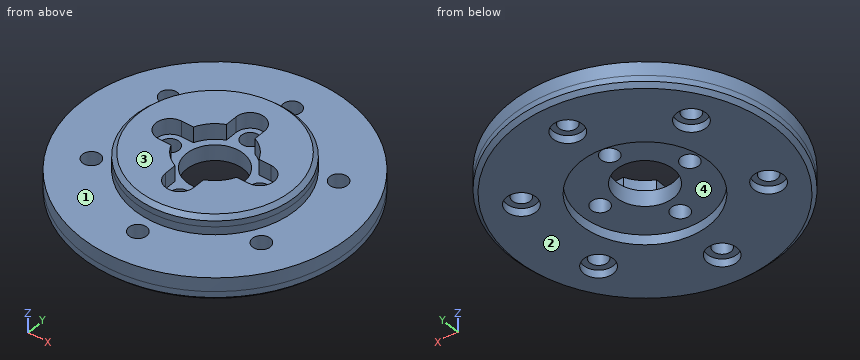
from build123d import *
from build123d.topology import SkipClean

# Parameters (mm, degrees)
SKETCH1_R               = 34.1
BOSS_EXTRUDE1_DEPTH     = 1.75
SKETCH4_R               = 28.5
BOSS_EXTRUDE2_DEPTH     = 2
SKETCH5_R               = 34.1
SKETCH5_R_2             = 16.25
BOSS_EXTRUDE3_DEPTH     = 2.5
CUT_EXTRUDE2_DEPTH      = 49.596501932
CUT_EXTRUDE2_DEPTH_BACK = 49.596501932
SKETCH3_R               = 2.25
CUT_EXTRUDE1_DEPTH      = 49.596501932
CUT_EXTRUDE1_DEPTH_BACK = 49.596501932
SKETCH2_R               = 7.25
SKETCH7_R               = 20.5
SKETCH7_R_2             = 2.25
SKETCH7_R_3             = 7.25
BOSS_EXTRUDE4_DEPTH     = 2.5
BOSS_EXTRUDE5_START     = 2
SKETCH8_R               = 34.1
SKETCH8_R_2             = 28.5
BOSS_EXTRUDE5_DEPTH     = 2
SKETCH10_R              = 34.1
SKETCH10_R_2            = 20.5
CUT_EXTRUDE4_DEPTH      = 2
CUT_EXTRUDE5_DEPTH      = 4
SKETCH6_R               = 2.25
CUT_EXTRUDE3_DEPTH      = 50.354533733
SKETCH12_R              = 3.75
CUT_EXTRUDE6_DEPTH      = 2
CIRPATTERN1_COUNT       = 6
CHAMFER1_SIZE           = 1


with BuildPart() as part:
    # Sketch1 → Boss-Extrude1 (new, symmetric)
    with BuildSketch(Plane.XY):
        Circle(SKETCH1_R)
    extrude(amount=BOSS_EXTRUDE1_DEPTH, both=True)

    # Sketch4 → Boss-Extrude2 (add)
    with BuildSketch(Plane.XY.offset(1.75)):
        Circle(SKETCH4_R)
    extrude(amount=BOSS_EXTRUDE2_DEPTH)

    # Sketch5 → Boss-Extrude3 (add)
    with BuildSketch(Plane(origin=(0, 0, -1.75), x_dir=(-1, 0, 0), z_dir=(0, 0, -1))):
        Circle(SKETCH5_R)
        Circle(SKETCH5_R_2, mode=Mode.SUBTRACT)
    extrude(amount=BOSS_EXTRUDE3_DEPTH)

    # Sketch3 → Cut-Extrude2 (cut, two sides: drawn at the far end of the back side and taken through both)
    with BuildSketch(Plane.XY.offset(1.75).offset(-CUT_EXTRUDE2_DEPTH_BACK)):
        with Locations((0, 11.3137085)):
            Circle(SKETCH3_R)
        with Locations((11.3137085, 0)):
            Circle(SKETCH3_R)
        with Locations((0, -11.3137085)):
            Circle(SKETCH3_R)
        with Locations((-11.3137085, 0)):
            Circle(SKETCH3_R)
    extrude(amount=CUT_EXTRUDE2_DEPTH + CUT_EXTRUDE2_DEPTH_BACK, mode=Mode.SUBTRACT)

    # Sketch2 → Cut-Extrude1 (cut, two sides: drawn at the far end of the back side and taken through both)
    with BuildSketch(Plane.XY.offset(1.75).offset(-CUT_EXTRUDE1_DEPTH_BACK)):
        Circle(SKETCH2_R)
    extrude(amount=CUT_EXTRUDE1_DEPTH + CUT_EXTRUDE1_DEPTH_BACK, mode=Mode.SUBTRACT)

    # Sketch7 → Boss-Extrude4 (add)
    with BuildSketch(Plane.XY.offset(3.75)):
        Circle(SKETCH7_R)
        with Locations((0, -11.3137085)):
            Circle(SKETCH7_R_2, mode=Mode.SUBTRACT)
        with Locations((11.3137085, 0)):
            Circle(SKETCH7_R_2, mode=Mode.SUBTRACT)
        with Locations((0, 11.3137085)):
            Circle(SKETCH7_R_2, mode=Mode.SUBTRACT)
        with Locations((-11.3137085, 0)):
            Circle(SKETCH7_R_2, mode=Mode.SUBTRACT)
        Circle(SKETCH7_R_3, mode=Mode.SUBTRACT)
    extrude(amount=BOSS_EXTRUDE4_DEPTH)

    # Sketch8 → Boss-Extrude5 (add)
    with SkipClean():  # the faces are left unmerged after this step: merging them gives an invalid solid
        with BuildSketch(Plane.XY.offset(1.75).offset(BOSS_EXTRUDE5_START)):
            with Locations(Location((0, 0, 0), (0, 0, 180))):
                Circle(SKETCH8_R)
            Circle(SKETCH8_R_2, mode=Mode.SUBTRACT)
        extrude(amount=-BOSS_EXTRUDE5_DEPTH)

    # Sketch10 → Cut-Extrude4 (cut)
    with BuildSketch(Plane.XY.offset(3.75)):
        with Locations(Location((0, 0, 0), (0, 0, 180))):
            Circle(SKETCH10_R)
        Circle(SKETCH10_R_2, mode=Mode.SUBTRACT)
    extrude(amount=-CUT_EXTRUDE4_DEPTH, mode=Mode.SUBTRACT)

    # Sketch11 → Cut-Extrude5 (cut)
    with BuildSketch(Plane.XY.offset(6.25)):
        with BuildLine():
            Line((-11.3137085, 3.6), (-8.248636251, 3.6))
            ThreePointArc((-8.248636251, 3.6), (-6.363961031, 6.363961031), (-3.6, 8.248636251))
            Line((-3.6, 8.248636251), (-3.6, 11.3137085))
            ThreePointArc((-3.6, 11.3137085), (0, 14.9137085), (3.6, 11.3137085))
            Line((3.6, 11.3137085), (3.6, 8.248636251))
            ThreePointArc((3.6, 8.248636251), (6.363961031, 6.363961031), (8.248636251, 3.6))
            Line((8.248636251, 3.6), (11.3137085, 3.6))
            ThreePointArc((11.3137085, 3.6), (14.9137085, 0), (11.3137085, -3.6))
            Line((11.3137085, -3.6), (8.248636251, -3.6))
            ThreePointArc((8.248636251, -3.6), (6.363961031, -6.363961031), (3.6, -8.248636251))
            Line((3.6, -8.248636251), (3.6, -11.3137085))
            ThreePointArc((3.6, -11.3137085), (0, -14.9137085), (-3.6, -11.3137085))
            Line((-3.6, -11.3137085), (-3.6, -8.248636251))
            ThreePointArc((-3.6, -8.248636251), (-6.363961031, -6.363961031), (-8.248636251, -3.6))
            Line((-8.248636251, -3.6), (-11.3137085, -3.6))
            ThreePointArc((-11.3137085, -3.6), (-14.9137085, 0), (-11.3137085, 3.6))
        make_face()
    extrude(amount=-CUT_EXTRUDE5_DEPTH, mode=Mode.SUBTRACT)

    # Sketch6 → Cut-Extrude3 (cut, symmetric)
    with BuildSketch(Plane.XY.offset(-4.25)):
        with Locations((0, 24.75)):
            Circle(SKETCH6_R)
    cut_extrude3 = extrude(amount=CUT_EXTRUDE3_DEPTH, both=True, mode=Mode.SUBTRACT)

    # Sketch12 → Cut-Extrude6 (cut)
    with BuildSketch(Plane(origin=(0, 0, -4.25), x_dir=(-1, 0, 0), z_dir=(0, 0, -1))):
        with Locations((0, 24.75)):
            Circle(SKETCH12_R)
    cut_extrude6 = extrude(amount=-CUT_EXTRUDE6_DEPTH, mode=Mode.SUBTRACT)

    # CirPattern1: Cut-Extrude3, Cut-Extrude6 ×6 about axis
    cirpattern1_axis = Axis((0, 0, 0), (0, 0, 1))
    add([cut_extrude3.rotate(cirpattern1_axis, i * 360 / CIRPATTERN1_COUNT) for i in range(1, CIRPATTERN1_COUNT)], mode=Mode.SUBTRACT)
    add([cut_extrude6.rotate(cirpattern1_axis, i * 360 / CIRPATTERN1_COUNT) for i in range(1, CIRPATTERN1_COUNT)], mode=Mode.SUBTRACT)

    # Chamfer1
    chamfer1_edges = [part.edges().sort_by_distance(p)[0] for p in [
        (34.1, 0, -4.25),
        (-20.5, 0, 6.25),
    ]]
    chamfer(chamfer1_edges, length=CHAMFER1_SIZE)


solid = part.part
Could you check a few things on this model? Use its own coordinates, in mm. Face numbers are marked on the shaded views. A direction names the side the tool comes from. Give positions to 0.01 mm unless a question says otherwise; leave off trailing zeros. Return JSON: item names as keys, results as strings.
1. I need wall thicknesses on line 1 (Y direction, x = 0, z = 1.2); line 2 (X direction, y = 11, z = -1.25); line 3 (Z direction, x = -13.5, y = 17.5). Which ranges of each line are inside material? Lowest first, please. Write a range as from..to.
Answer list:
{"line 1": "y = -34.1..-27, -22.5..-13.56, -9.06..-7.25, 7.25..9.06, 13.56..22.5, 27..34.1", "line 2": "x = -32.28..-23.22, -19.65..-2.23, 2.23..19.65, 23.22..32.28", "line 3": "z = -4.25..1.75"}
2. Imagine slicing it at A-A on y = 0. Give the number of separate pieces and of enclosed holes in the cut face, then the cut area to 3 significant figures.
Answer list:
{"separate pieces": "4", "enclosed holes": "0", "area": "297 mm2"}
3. On a 3-axis mill with a long thin cutter (end or side, diameter ignored), from which of +Z, -Z, +X, -X, +Y, -Y can I reach the whole of each face in a straight line? I mean the marked faces 1 and 2. Say none if no direction works.
Answer list:
{"face 1": "+Z", "face 2": "-Z, +X, -X, +Y, -Y"}
4. Thinking about a two-plate mould opening in Y: for the marked faces 3 and 4, which applies, pulls with the +Y half, pulls with the -Y half, needs draft (parallel to the pull), parting line crosses it, or undercut?
Answer list:
{"face 3": "needs draft", "face 4": "undercut"}
5. For pin 1 Ø3.5 at (y, z) = (-9.5, 5) entering from +X; pin 2 Ø6 at (x, y) = (22, 25.5) entering from -Z; pin 3 Ø6 at (x, y) = (-21.5, -12.5) entering from -Z; pin 4 Ø6 at (x, z) = (-26.5, -3) entering from -Y, each with a flat end and sliding along its axis, tell me the tip position at first contact or that it passes through.
Answer list:
{"pin 1": "stops at x = 18.98", "pin 2": "stops at z = -4.25", "pin 3": "stops at z = -2.25", "pin 4": "stops at y = -24.71"}
